For this review, take the finished solid that the model builds, in its own axes (mm). Give positions to 0.01 mm unless a question says otherwise; leave off trailing zeros. Order: outer loops, then holes, each group sorted by start corner. A loop starts at its lowest first (then second) coordinate and runs counter-clockwise, first axis right, second up. Notation, with made-up numbers: (81.5, 49.25) -> (137.5, 49.25) arc R5 ccw to (137.5, 54.25) -> close; hole circle Ø7 at (80, -13.75). An arc over 180 degrees is marked (long way). Use CSV: the item, a comma, the result in double quotes. Start each with the question number.
```python
from build123d import *

# Parameters (mm, degrees)
SKETCH1_W           = 25.06
SKETCH1_H           = 17.41
BOSS_EXTRUDE1_DEPTH = 0.75
FILLET4_R           = 0.5
SKETCH2_W           = 23.06
SKETCH2_H           = 16.41
CUT_EXTRUDE1_DEPTH  = 0.25
SCALE1_SCALE        = 10


with BuildPart() as part:
    # Sketch1 → Boss-Extrude1 (new body)
    with BuildSketch(Plane(origin=(0, 0, 0), x_dir=(0, 0, -1), z_dir=(1, 0, 0))):
        Rectangle(SKETCH1_W, SKETCH1_H)
    extrude(amount=BOSS_EXTRUDE1_DEPTH)

    # Fillet4
    fillet4_edges = [part.edges().sort_by_distance(p)[0] for p in [
        (0, -8.705, 0),
        (0, 0, 12.53),
        (0, 8.705, 0),
        (0, 0, -12.53),
    ]]
    fillet(fillet4_edges, radius=FILLET4_R)

    # Sketch2 → Cut-Extrude1 (cut)
    with BuildSketch(Plane(origin=(0.75, 0, 0), x_dir=(0, 0, -1), z_dir=(1, 0, 0))):
        Rectangle(SKETCH2_W, SKETCH2_H)
    extrude(amount=-CUT_EXTRUDE1_DEPTH, mode=Mode.SUBTRACT)


with BuildPart() as part_1:
    # Scale1: scaled about (0.276512494, 0, 0)
    add(part.part.scale(SCALE1_SCALE).moved(Location((-2.488612446, 0, 0))))


solid = part_1.part
```
1. Draft analysis for pull direction Z (two halves, no side actions). For faces 1 (the face through (-0.99, 1.22, -123.87)), 2 (the face through (2.511, 1, 2)), 3 (the face through (5.011, -83, 10)), 4 (the face through (-0.99, 1.22, 123.87)), state which applies: +Z half, -Z half, draft (parallel to the pull), parting line (faces both ways), or undercut.
2. To check wall thickness, follow L1, parallel to Z at x = 3.25, y = 6; L2, parallel to Y at x = 4, z = 49; L3, parallel to X at y = -58, z = 102. State the ranges of each line that lie inside material, in increasing order. Write a range as [from, to].
3. Consider section B-B (z = -103.5). State the section outline as (x, y) points.
4. Consider section A-A (y = 6). State the section outline as (x, z) points, plus the area to 3 significant figures.
5. Consider section C-C (x = -0.5). State the section outline as (y, z) points, plus the area to 3 significant figures.
6. Clearance check with flat-ended pins moving along their axes: P1, Ø8, axis at y = 24, z = 68, coming from the +X side; P2, Ø1, axis at x = 0, z = -90, coming from the +Y side. State where each tip first meets the part, or that it passes through.
Answer list:
1,face 1,"-Z half"
1,face 2,"undercut"
1,face 3,"draft"
1,face 4,"+Z half"
2,L1,"[-125.3, -115.3], [115.3, 125.3]"
2,L2,"[-87.05, -82.05], [82.05, 87.05]"
2,L3,"[-2.49, 2.51]"
3,outline,"(-2.49, -82.05) arc R5 ccw to (2.51, -87.05) -> (5.01, -87.05) -> (5.01, -82.05) -> (2.51, -82.05) -> (2.51, 82.05) -> (5.01, 82.05) -> (5.01, 87.05) -> (2.51, 87.05) arc R5 ccw to (-2.49, 82.05) -> close"
4,outline,"(-2.49, -120.3) arc R5 ccw to (2.51, -125.3) -> (5.01, -125.3) -> (5.01, -115.3) -> (2.51, -115.3) -> (2.51, 115.3) -> (5.01, 115.3) -> (5.01, 125.3) -> (2.51, 125.3) arc R5 ccw to (-2.49, 120.3) -> close"
4,area,"1,290 mm2"
5,outline,"(-86.04, -124.29) -> (86.04, -124.29) -> (86.04, 124.29) -> (-86.04, 124.29) -> close"
5,area,"42,800 mm2"
6,P1,"x = 2.51"
6,P2,"y = 86.63"
